Source: CAD feature listing. Evaluate the final solid. Frame: model axes, mm. A direction names the side the tool comes from. Round coordinates to 2 decimals unless told otherwise and drop trailing zeros. Write each loop counter-clockwise with the first axis right and the second up, starting at its lowest first coordinate (ties: lowest second). Pieces come first, ordered by that corner, then holes. Notation, with made-up numbers: (-22, -6.75) -> (-17, -6.75) arc R10 ccw to (-17, -2.75) -> close; hole circle Ø2 at (-3.75, 27). An arc over 180 degrees is marked (long way). Put each result on its own line as item: value.
```python
from build123d import *

# Parameters (mm, degrees)
SKETCH1_W           = 10
SKETCH1_H           = 27.05
SKETCH1_R           = 1
SKETCH1_H_2         = 3.25
BOSS_EXTRUDE1_DEPTH = 15
SKETCH2_OUTSIDE_W   = 19.052
SKETCH2_OUTSIDE_H   = 39.352
SKETCH2_OUTSIDE_W_2 = 10
SKETCH2_OUTSIDE_H_2 = 10
CUT_EXTRUDE1_DEPTH  = 2


with BuildPart() as part:
    # Sketch1 → Boss-Extrude1 (new body)
    with BuildSketch(Plane.XY):
        with Locations((0, 9.525)):
            Rectangle(SKETCH1_W, SKETCH1_H)
        with Locations((0, 19.05)):
            Circle(SKETCH1_R, mode=Mode.SUBTRACT)
        Circle(SKETCH1_R, mode=Mode.SUBTRACT)
        with Locations((0, -5.625)):
            Rectangle(SKETCH1_W, SKETCH1_H_2)
    extrude(amount=-BOSS_EXTRUDE1_DEPTH)

    # Sketch2 outside → Cut-Extrude1 (cut)
    with BuildSketch(Plane.XY):
        with Locations((0, 7.9)):
            Rectangle(SKETCH2_OUTSIDE_W, SKETCH2_OUTSIDE_H)
        with Locations((0, 19.05)):
            Rectangle(SKETCH2_OUTSIDE_W_2, SKETCH2_OUTSIDE_H_2, mode=Mode.SUBTRACT)
        Rectangle(SKETCH2_OUTSIDE_W_2, SKETCH2_OUTSIDE_H_2, mode=Mode.SUBTRACT)
    extrude(amount=-CUT_EXTRUDE1_DEPTH, mode=Mode.SUBTRACT)


solid = part.part
```
Q1. Cut plane B-B on x = 0. Output: boundary loops of the cut face in (y, z).
Ans:
outline: (-7.25, -15) -> (-1, -15) -> (-1, 0) -> (-5, 0) -> (-5, -2) -> (-7.25, -2) -> close; (1, -15) -> (18.05, -15) -> (18.05, 0) -> (14.05, 0) -> (14.05, -2) -> (5, -2) -> (5, 0) -> (1, 0) -> close; (20.05, -15) -> (23.05, -15) -> (23.05, 0) -> (20.05, 0) -> close
Q2. Material intervals for line 1 (Y direction, x = 0, z = -5.5); line 2 (Y direction, x = -3.5, z = -1); line 3 (Z direction, x = 3.5, y = 13), sorted ascending. Write a range as [from, to].
Ans:
line 1: y = [-7.25, -1], [1, 18.05], [20.05, 23.05]
line 2: y = [-5, 5], [14.05, 23.05]
line 3: z = [-15, -2]
Q3. Cut plane D-D on x = -3. Output: boundary loops of the cut face in (y, z), and give its area (3 significant figures).
Ans:
outline: (-7.25, -15) -> (23.05, -15) -> (23.05, 0) -> (14.05, 0) -> (14.05, -2) -> (5, -2) -> (5, 0) -> (-5, 0) -> (-5, -2) -> (-7.25, -2) -> close
area: 432 mm^2
Q4. Draft query along Y for faces 1 (the flat face through (0, 5, -1)), 2 (the flat face through (0, -5, -1)), 3 (the flat face through (-5, 8, -7)), 4 (the flat face through (0, 23.05, -7)). Return one class per face: +Y half, -Y half, draft (parallel to the pull), parting line (faces both ways), or undercut.
Ans:
face 1: undercut
face 2: -Y half
face 3: draft
face 4: +Y half
Q5. Pin query (flat end, axial travel): pin 1 (1.1 mm diameter, centred on x = -2, y = -6, fed in from +Z); pin 2 (0.6 mm diameter, centred on x = 0.5, z = -1, fed in from -Y). Return the tip coordinate at first contact, or that it passes through.
Ans:
pin 1: stops at z = -2
pin 2: stops at y = -5
Q6. Reachability of faces 5 (the flat face through (-0.1, 17.6, 0)), 6 (the flat face through (0, -6, -2)), 7 (the flat face through (0, 14.05, -1)) from +Z, -Z, +X, -X, +Y, -Y: full face, straight path, thin tool, end or side. Return the list, or none.
Ans:
face 5: +Z, +X, -X, +Y, -Y
face 6: +Z, +X, -X, -Y
face 7: +Z, +X, -X
Q7. Cut plane A-A on y = 19.05. Output: boundary loops of the cut face in (x, z), and give its area (3 significant figures).
Ans:
outline: (-5, -15) -> (-1, -15) -> (-1, 0) -> (-5, 0) -> close; (1, -15) -> (5, -15) -> (5, 0) -> (1, 0) -> close
area: 120 mm^2
Q8. Cut plane C-C on z = -4.5. Output: boundary loops of the cut face in (x, y).
Ans:
outline: (-5, -7.25) -> (5, -7.25) -> (5, 23.05) -> (-5, 23.05) -> close; hole circle Ø2 at (0, 0); hole circle Ø2 at (0, 19.05)
